from build123d import *

# Parameters (mm, degrees)
POCKET001_DEPTH       = 54.489273
POCKET001_DEPTH_BACK  = 86.48894
POLARPATTERN001_COUNT = 5


with BuildPart() as part:
    # Sketch024 → Revolution001 (revolve)
    with BuildSketch(Plane.YZ):
        with BuildLine():
            Line((-31.999667, 8.950126), (-30.949667, 8.950126))
            Line((-30.949667, 7.950126), (-30.949667, 8.950126))
            Line((-22.929667, 7.950126), (-30.949667, 7.950126))
            Line((-22.929667, 8.950126), (-22.929667, 7.950126))
            Line((-22.929667, 8.950126), (-21.929667, 8.950126))
            Line((-21.929667, 8.950126), (-21.929667, 7.950126))
            ThreePointArc((-22.929667, 6.950126), (-22.225454, 7.245913), (-21.929667, 7.950126))
            Line((-22.929667, 6.950126), (-24.999667, 6.950126))
            ThreePointArc((-24.999667, 6.950126), (-25.699738, 6.655996), (-25.979667, 5.950126))
            Line((-25.979667, 2.4), (-25.979667, 5.950126))
            Line((-28.779667, 2.4), (-25.979667, 2.4))
            Line((-28.779667, 0.8), (-28.779667, 2.4))
            Line((-30.379667, 0.8), (-28.779667, 0.8))
            Line((-30.379667, 1.7), (-30.379667, 0.8))
            Line((-31.999667, 1.7), (-30.379667, 1.7))
            Line((-31.999667, 8.950126), (-31.999667, 1.7))
        make_face()
    revolve(axis=Axis((0, 0, 0), (0, 1, 0)))

    # Sketch025 → Pocket001 (cut, two sides)
    with BuildSketch(Plane(origin=(-5.2, 0, 0), x_dir=(1, 0, 0), z_dir=(0, -1, 0))) as pocket001_sk:
        with BuildLine():
            add(Edge.make_bspline(
                [(7.722002, 5.067158), (5.222002, 0.076099), (2.722002, 5.067158)],
                knots=[-2.5, -2.5, -2.5, 2.5, 2.5, 2.5], degree=2))
            ThreePointArc((2.722002, 5.067158), (5.222002, 5.573306), (7.722002, 5.067158))
        make_face()
    pocket001 = extrude(amount=-POCKET001_DEPTH, mode=Mode.SUBTRACT) + extrude(pocket001_sk.sketch, amount=POCKET001_DEPTH_BACK, mode=Mode.SUBTRACT)

    # PolarPattern001: Pocket001 ×5 about axis
    polarpattern001_axis = Axis((0, 0, 0), (0, 1, 0))
    for i in range(1, POLARPATTERN001_COUNT):
        add(pocket001.rotate(polarpattern001_axis, i * 360 / POLARPATTERN001_COUNT), mode=Mode.SUBTRACT)


with BuildPart() as part_1:
    # Body021 placement: moved
    add(part.part.moved(Location((54.7, 7, -10.5))))


solid = part_1.part
Geometry check sheet. Reference: the model listing, model coordinates, mm. A direction names the side the tool comes from. Round coordinates to 2 decimals unless told otherwise and drop trailing zeros. Answer in a Markdown table with one row per item. Add a question column.
Item 1: Set-up check for faces 4 (the face through (59.996, -22.032, -8.765)), 5 (the face through (57.08, -20.36, -10.81)), 6 (the face through (46.94, -20, -12.22)), 7 (the face through (53.04, -24.18, -10.87)): record each of +Z, -Z, +X, -X, +Y, -Y from which the full face is reachable in a straight line by a thin tool's end or side.
Item 2: Sectioned sample at A-A, the plane z = -14.5. State how many separate pieces and enclosed holes the cut face has, plus the area to 3 significant figures.
Item 3: Draft check along X on faces 1 (the face through (45.963, -24.467, -12.44)), 2 (the face through (63, -15.93, -11)), 3 (the face through (49.395, -22.032, -8.791)). Enter one of: released by +X, released by -X, zero draft, split by the parting line, or undercut.
Item 4: Depth check by flat-ended pin: pin 1 Ø2 at (x, z) = (54.5, -15) entering from +Y; pin 2 Ø2.5 at (x, z) = (54.7, -10.5) entering from -Y; pin 3 Ø4 at (y, z) = (-20, -13.5) entering from -X. Enter the tip coordinate at first touch or a pass-through.
Item 5: Material ranges on L1, parallel to Z at x = 54.75, y = -19.75; L2, parallel to Y at x = 46.5, z = -7.5; L3, parallel to X at y = -24, z = -8.75, recorded low to high. Write a range as [from, to].
Filled in:
| question | item | result |
|---|---|---|
| 1 | face 4 | +Y, -Y |
| 1 | face 5 | +Y |
| 1 | face 6 | none |
| 1 | face 7 | -Y |
| 2 | separate pieces | 3 |
| 2 | enclosed holes | 0 |
| 2 | area | 59.9 mm² |
| 3 | face 1 | split by the parting line |
| 3 | face 2 | zero draft |
| 3 | face 3 | undercut |
| 4 | pin 1 | stops at y = -18.98 |
| 4 | pin 2 | stops at y = -23.38 |
| 4 | pin 3 | stops at x = 46.81 |
| 5 | L1 | z = [-18.45, -12.9], [-8.1, -7.93], [-4.93, -2.55] |
| 5 | L2 | y = [-25, -23.95], [-15.93, -14.93] |
| 5 | L3 | x = [45.92, 49.41], [52.24, 57.19], [59.99, 63.48] |
